For this review, take the finished solid that the model builds, in its own axes (mm). Face numbers are marked on the shaded views. A direction names the side the tool comes from. Coordinates: 2 decimals unless noted, no trailing zeros. Write each loop counter-clockwise with the first axis right and the second up, starting at its lowest first coordinate (ties: lowest second). Pieces come first, ordered by that corner, then holes. Notation, with made-up numbers: (59.25, 45) -> (115.25, 45) arc R15 ccw to (115.25, 54) -> close; hole circle Ø5 at (14, 39). An arc over 180 degrees is marked (long way). One line per item, written item: value. Start each with the question number.
1) Add section A-A (z = -44.5). State the section outline as (x, y) points, and give its area (3 significant figures).
2) For probe 1 along Z at (x, y) = (-10, -3.25); probe 2 along Z at (x, y) = (-22.5, 4); probe 3 along Z at (x, y) = (-17.75, -0.5), list the stretches that pass through material, from the lowest coordinate up. Write a range as from..to.
3) Mouldability with a two-part tool opening along Y and no side actions: class the marked faces 4, 5 and 6 as released by +Y, released by -Y, zero draft, split by the parting line, or undercut.
4) Add section D-D (y = -1.5). State how many separate pieces and enclosed holes the cut face has, and give its area (3 significant figures).
5) Add section B-B (x = -17.5). State the section outline as (y, z) points, and give its area (3 significant figures).
6) Machinability: for the marked faces 1, 2 and 3, which of the approach directions +Z, -Z, +X, -X, +Y, -Y give a long, thin tool a straight path to every point of the face, cutting with its end or side? Answer none if there is none.
7) For pin 1 Ø5.5 at (x, z) = (-5.5, -21.5) entering from +Y; pin 2 Ø1.6 at (y, z) = (-0.5, -19.5) entering from +X; pin 3 Ø1 at (y, z) = (0, -20) entering from -X; pin 4 Ø1.6 at (y, z) = (0, -20) entering from +X, all flat-tipped, find the tip position at first contact; note any pin that passes through.
8) Add section C-C (z = -7). State the section outline as (x, y) points.
Autodesk Inventor part; units mm, degrees
ref_plane "YZ Plane" through (0, 0, 0) normal (1, 0, 0) x (0, 1, 0)
ref_plane "XZ Plane" through (0, 0, 0) normal (0, 1, 0) x (-1, 0, 0)
ref_plane "XY Plane" through (0, 0, 0) normal (0, 0, 1) x (1, 0, 0)
sketch "Sketch1" plane through (0, 0, 0) normal (0, 1, 0) x (-1, 0, 0)
  line L0 (24.505382, -20) -> (6.505382, -20) construction
  line L1 (6.505382, -20) -> (6.505382, -29.5) construction
  line L2 (6.505382, -29.5) -> (24.505382, -29.5) construction
  line L3 (0, -36.005382) -> (10.505382, -25.5)
  line L4 (11.313708, -13.494618) -> (0, -24.808326)
  line L5 (8.505382, -18) -> (0, -26.505382)
  line L6 (8.505382, -18) -> (10.505382, -18)
  line L7 (0, 0) -> (24.505382, 0)
  line L8 (24.505382, 0) -> (24.505382, -49.5)
  line L9 (24.505382, -49.5) -> (0, -49.5)
  line L10 (0, -49.5) -> (0, 0)
  line L11 (6.505382, -20) -> (5.656854, -19.151472) construction
  line L12 (10.505382, -18) -> (10.505382, -25.5)
  line L13 (11.313708, -13.494618) -> (11.313708, 0)
  line L14 (2.727208, -33.278175) -> (5.06066, -35.611627)
  line L15 (5.06066, -35.611627) -> (14.253048, -26.419239)
  line L16 (14.253048, -26.419239) -> (11.919596, -24.085786)
  line L17 (7.323402, -28.681981) -> (9.656854, -31.015433)
  line L18 (10.505382, -25.5) -> (11.919596, -24.085786)
  line L19 (3.434315, -32.571068) -> (2.868629, -32.005382)
  line L20 (2.868629, -32.005382) -> (0, -34.874012)
  circle A0 centre (8.490128, -29.848707) radius 1
  line L21 (24.505382, -20) -> (10.505382, -20)
  line L22 (24.505382, -22) -> (18.505382, -22)
  line L23 (18.505382, -22) -> (18.505382, -20.6)
  line L24 (18.505382, -20.6) -> (15.505382, -20.6)
  line L25 (15.505382, -20.6) -> (15.505382, -21)
  line L26 (15.505382, -21) -> (10.505382, -21)
  dimension "d0" = 45
  dimension "d1" = 45
  dimension "d2" = 1.2
  dimension "d3" = 2
  dimension "d4" = 14
  dimension "d5" = 8
  dimension "d6" = 8
  dimension "d9" = 20
  dimension "d10" = 20
  dimension "d11" = 9.5
  dimension "d12" = 3.3
  dimension "d13" = 13
  dimension "d14" = 2
  dimension "d46" = 2
  dimension "d49" = 0.8
  dimension "d50" = 1
  dimension "d51" = 2
  dimension "d52" = 1
  dimension "d53" = 0.6
  dimension "d54" = 5
  dimension "d55" = 6
  dimension "d56" = 2
extrude "Extrusion1" add sketch "Sketch1" along normal blind 8 and the other way blind 10 contours L10 L20 L19 L3 | L3 L14 L15 L16 L18 L12 L26 L25 L24 L23 L22 L8 L9 L10 | L3 L17 A0 L15 L14 | L10 L5 L6 L12 L3 L19 L20 | L10 L4 L13 L7 L8 L21 L12 L6 L5 | L3 L18 L16 L15 L17 A0 | L22 L23 L24 L25 L26 L12 L21 L8 | L10 L7 L13 L4
extrude "Extrusion2" cut sketch "Sketch1" along normal blind 13 and the other way blind 8 contours L10 L5 L6 L12 L3 L19 L20 | L10 L7 L13 L4
revolve "Revolution2" cut sketch "Sketch1" angle 360 about axis through (-24.505382, 0, -20) along (1, 0, 0) contours L22 L23 L24 L25 L26 L12 L21 L8
extrude "Extrusion3" cut sketch "Sketch1" along normal blind 13 contours L3 L17 A0 L15 L14 | L3 L18 L16 L15 L17 A0 | A0 L17 | L17 A0
revolve "Revolution1" cut sketch "Sketch1" angle 360 about axis through (-7.323402, 0, -28.681981) along (-0.7071068, 0, -0.7071068) picked at (8.589296, -30.166947) contours L3 L17 A0 L15 L14 | L17 A0
sketch "Sketch2" plane through (-24.505382, -10, 0) normal (-1, 0, 0) x (0, 0, 1)
  line L0 (-33.75, 5.75) -> (-25.25, 5.75)
  line L1 (-25.25, 5.75) -> (-25.25, 14.25)
  line L2 (-25.25, 14.25) -> (-33.75, 14.25)
  line L3 (-33.75, 14.25) -> (-33.75, 5.75)
  circle A0 centre (-20, 10) radius 1
  circle A1 centre (-20, 10) radius 2
  circle A2 centre (-44.5, 8) radius 1.397
  circle A3 centre (-4.5, 8) radius 1.397
  point P0 (0, 10)
  point P1 (-20, 10)
  point P2 (-20, 10)
  point P3 (-20, 10)
  point P4 (-29.5, 10)
  point P5 (-29.5, 10)
  point P6 (-29.5, 10)
  point P7 (-33.75, 10)
  point P8 (-29.5, 14.25)
  dimension "d24" = 8.5
  dimension "d25" = 15.5
  dimension "d26" = 2
  dimension "d27" = 2.794
  dimension "d28" = 15
  dimension "d29" = 4
  dimension "d30" = 2
extrude "Extrusion4" cut sketch "Sketch2" against normal up to next contours L3 L2 L1 L0 | A2 | A3
sketch "Sketch3" plane through (-11.313708, -8, -13.494618) normal (0.7071068, 0, 0.7071068) x (0.7071068, 0, -0.7071068)
  line L0 (2, 2) -> (14, 2) construction
  line L1 (14, 2) -> (14, 14) construction
  line L2 (14, 14) -> (2, 14) construction
  line L3 (2, 14) -> (2, 2) construction
  line L4 (3.5, 3.5) -> (19.455942, 3.5)
  line L5 (19.455942, 3.5) -> (19.455942, 23.765103)
  line L6 (19.455942, 23.765103) -> (3.5, 23.765103)
  line L7 (3.5, 23.765103) -> (3.5, 3.5)
  circle A0 centre (2, 2) radius 0.6
  circle A1 centre (2, 14) radius 0.6
  circle A2 centre (14, 2) radius 0.6
  point P0 (-1.542136, 8)
  point P1 (8, 8)
  point P2 (8, 8)
  point P3 (8, 8)
  point P4 (14, 8)
  point P5 (8, 14)
  dimension "d35" = 4.5
  dimension "d36" = 4.5
  dimension "d37" = 12
  dimension "d38" = 1.2
extrude "Extrusion6" cut sketch "Sketch3" against normal blind 2.7 contours L7 L6 L5 L4
extrude "Extrusion7" cut sketch "Sketch3" against normal blind 7 contours A0 | A1 | A2
chamfer "Chamfer1" distance 1.27 angle 45 4 edges at (-12.2527, -10, -49.5) (0, -10, -24.75) (-24.5054, -10, -24.75) (-12.2527, -10, 0)
properties part number "minimal micro scanner 2"
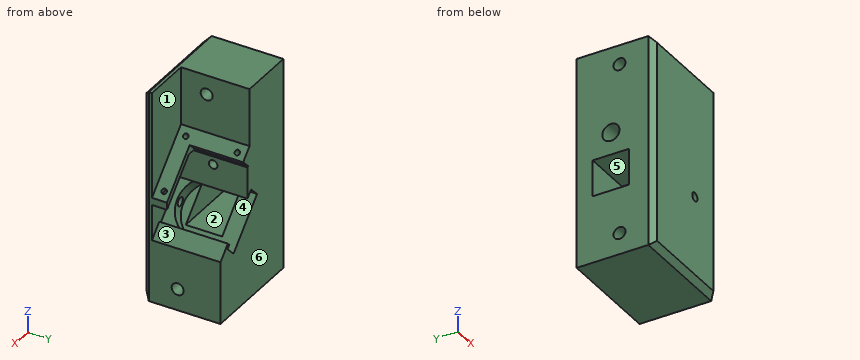
Numbers:
1. outline: (-24.51, -8.73) -> (-23.24, -10) -> (-1.27, -10) -> (0, -8.73) -> (0, -3.4) -> (-24.51, -3.4) -> close; (-24.51, -0.6) -> (0, -0.6) -> (0, 8) -> (-24.51, 8) -> close
1. area: 371 mm²
2. probe 1: -49.5..-45.12, -43.88..-33.75, -17.13..-14.81
2. probe 2: -49.5..-33.75, -25.25..0
2. probe 3: -49.5..-33.75, -25.25..-20.33, -19.67..0
3. face 4: zero draft
3. face 5: undercut
3. face 6: released by +Y
4. separate pieces: 4
4. enclosed holes: 0
4. area: 614 mm²
5. outline: (-10, -48.23) -> (-8.73, -49.5) -> (8, -49.5) -> (8, 0) -> (-8.73, 0) -> (-10, -1.27) -> close; hole (-4.25, -33.75) -> (4.25, -33.75) -> (4.25, -25.25) -> (-4.25, -25.25) -> close; hole circle Ø2.79 at (-2, -44.5); hole circle Ø2.79 at (-2, -4.5); hole circle Ø1.2 at (0, -20)
5. area: 804 mm²
6. face 1: +Z, +X, +Y
6. face 2: -X
6. face 3: +X, +Y
7. pin 1: y = -4.5
7. pin 2: x = -10.51
7. pin 3: through
7. pin 4: x = -15.51
8. outline: (-24.51, -8.73) -> (-23.24, -10) -> (-1.27, -10) -> (0, -8.73) -> (0, -8) -> (-11.31, -8) -> (-11.31, 8) -> (-24.51, 8) -> close
